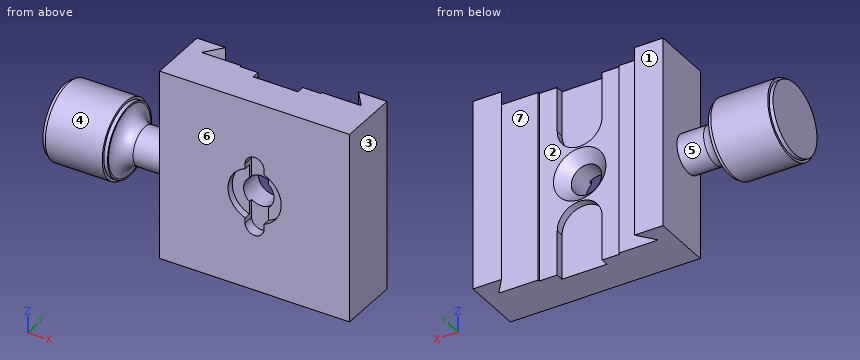
from build123d import *

# Parameters (mm, degrees)
SKETCH_1_R          = 5.9
EXTRUDE_1_DEPTH     = 8.94
SKETCH_1_4_R        = 4
EXTRUDE_2_DEPTH     = 11
SKETCH_1_5_W        = 14.4
SKETCH_1_5_H        = 50
EXTRUDE_3_DEPTH     = 16
CUT_EXTRUDE_1_DEPTH = 59.14636704
SKETCH_4_R          = 5
EXTRUDE_4_DEPTH     = 11
SKETCH_5_R          = 9.4
EXTRUDE_5_DEPTH     = 1
SKETCH_6_R          = 10.05
EXTRUDE_6_DEPTH     = 15
SKETCH_7_R          = 9.4
EXTRUDE_7_DEPTH     = 1
FILLET_1_R          = 4
CUT_EXTRUDE_3_DEPTH = 1.8
CUT_EXTRUDE_4_DEPTH = 2.8


with BuildPart() as part:
    # 草图1 → 凸台-拉伸1 (new body)
    with BuildSketch(Plane(origin=(0, 0, 0), x_dir=(1, 0, 0), z_dir=(0, 1, 0))):
        with BuildLine():
            Line((-5.9, -13.2), (-5.9, -25))
            Line((-5.9, -25), (5.9, -25))
            Line((5.9, -25), (5.9, -13.2))
            ThreePointArc((5.9, -13.2), (0, -19.1), (-5.9, -13.2))
        make_face()
        with Locations((0, -13.2)):
            Circle(SKETCH_1_R)
        with Locations((0, 13.2)):
            Circle(SKETCH_1_R)
        with BuildLine():
            Line((-5.9, 25), (-5.9, 13.2))
            ThreePointArc((-5.9, 13.2), (0, 19.1), (5.9, 13.2))
            Line((5.9, 13.2), (5.9, 25))
            Line((5.9, 25), (-5.9, 25))
        make_face()
    extrude(amount=EXTRUDE_1_DEPTH)

    # 草图1<4> → 凸台-拉伸2 (add)
    with BuildSketch(Plane(origin=(0, 0, 0), x_dir=(1, 0, 0), z_dir=(0, 1, 0))):
        with BuildLine():
            ThreePointArc((5.9, 13.2), (0, 7.3), (-5.9, 13.2))
            Line((-5.9, 13.2), (-5.9, 25))
            Line((-5.9, 25), (-10.6, 25))
            Line((-10.6, 25), (-10.6, -25))
            Line((-10.6, -25), (-5.9, -25))
            Line((-5.9, -25), (-5.9, -13.2))
            ThreePointArc((-5.9, -13.2), (0, -7.3), (5.9, -13.2))
            Line((5.9, -13.2), (5.9, -25))
            Line((5.9, -25), (10.6, -25))
            Line((10.6, -25), (10.6, 25))
            Line((10.6, 25), (5.9, 25))
            Line((5.9, 25), (5.9, 13.2))
        make_face()
        with Locations(Location((0, 0, 0), (0, 0, 270))):
            Circle(SKETCH_1_4_R, mode=Mode.SUBTRACT)
    extrude(amount=EXTRUDE_2_DEPTH)

    # 草图1<5> → 凸台-拉伸3 (add)
    with BuildSketch(Plane(origin=(0, 0, 0), x_dir=(1, 0, 0), z_dir=(0, 1, 0))):
        with Locations((17.8, 0)):
            Rectangle(SKETCH_1_5_W, SKETCH_1_5_H)
        with Locations((-17.8, 0)):
            Rectangle(SKETCH_1_5_W, SKETCH_1_5_H)
    extrude(amount=EXTRUDE_3_DEPTH)

    # 草图2 → 切除-拉伸1 (cut, through all)
    with BuildSketch(Plane.XY.offset(25)):
        Polygon((-17.5, 16), (-21, 11.5), (21, 11.5), (17.5, 16), align=None)
    extrude(amount=-CUT_EXTRUDE_1_DEPTH, mode=Mode.SUBTRACT)

    # 切除-拉伸2 cone 1 section (through the dimple's axis) → 切除-拉伸2 (revolve, cut)
    with BuildSketch(Plane(origin=(0, 11, 0), x_dir=(0, 0, 1), z_dir=(1, 0, 0))):
        Polygon((0, 0), (6.9, 0), (0, 6.9), align=None)
    revolve(axis=Axis((0, 11, 0), (0, -1, 0)), mode=Mode.SUBTRACT)

    # 草图4 → 凸台-拉伸4 (add)
    with BuildSketch(Plane.ZY.offset(25)):
        with Locations(Location((0, 5, 0), (0, 0, 270))):
            Circle(SKETCH_4_R)
    extrude(amount=EXTRUDE_4_DEPTH)

    # 草图5 → 凸台-拉伸5 (add)
    with BuildSketch(Plane.ZY.offset(36)):
        with Locations((0, 5)):
            Circle(SKETCH_5_R)
    extrude(amount=EXTRUDE_5_DEPTH)

    # 草图6 → 凸台-拉伸6 (add)
    with BuildSketch(Plane.ZY.offset(37)):
        with Locations((0, 5)):
            Circle(SKETCH_6_R)
    extrude(amount=EXTRUDE_6_DEPTH)

    # 草图7 → 凸台-拉伸7 (add)
    with BuildSketch(Plane.ZY.offset(52)):
        with Locations((0, 5)):
            Circle(SKETCH_7_R)
    extrude(amount=EXTRUDE_7_DEPTH)

    # 圆角1
    fillet_1_edges = [part.edges().sort_by_distance(p)[0] for p in [
        (-36, 10, 0),
    ]]
    fillet(fillet_1_edges, radius=FILLET_1_R)

    # 草图8 → 切除-拉伸3 (cut)
    with BuildSketch(Plane.XZ):
        with BuildLine():
            Line((-2.5, 3.122498999), (-2.5, 6.538348415))
            ThreePointArc((-2.5, 6.538348415), (-7, 0), (-2.5, -6.538348415))
            Line((-2.5, -6.538348415), (-2.5, -3.122498999))
            ThreePointArc((-2.5, -3.122498999), (-4, 0), (-2.5, 3.122498999))
        make_face()
        with BuildLine():
            ThreePointArc((7, 0), (5.766281297, 3.968626967), (2.5, 6.538348415))
            Line((2.5, 6.538348415), (2.5, 3.122498999))
            ThreePointArc((2.5, 3.122498999), (3.605551275, 1.732050808), (4, 0))
            ThreePointArc((4, 0), (3.605551275, -1.732050808), (2.5, -3.122498999))
            Line((2.5, -3.122498999), (2.5, -6.538348415))
            ThreePointArc((2.5, -6.538348415), (5.766281297, -3.968626967), (7, 0))
        make_face()
    extrude(amount=-CUT_EXTRUDE_3_DEPTH, mode=Mode.SUBTRACT)

    # 草图8<3> → 切除-拉伸4 (cut)
    with BuildSketch(Plane.XZ):
        with BuildLine():
            Line((2.5, 7.9), (2.5, -7.9))
            ThreePointArc((2.5, -7.9), (0, -10.4), (-2.5, -7.9))
            Line((-2.5, -7.9), (-2.5, 7.9))
            ThreePointArc((-2.5, 7.9), (0, 10.4), (2.5, 7.9))
        make_face()
    extrude(amount=-CUT_EXTRUDE_4_DEPTH, mode=Mode.SUBTRACT)


solid = part.part
CAD build for the part. Positions are in the model's coordinates, mm. Face numbers are marked on the shaded views. A direction names the side the tool comes from. Give positions to 0.01 mm unless a question says otherwise; leave off trailing zeros. Write each loop counter-clockwise with the first axis right and the second up, starting at its lowest first coordinate (ties: lowest second). Pieces come first, ordered by that corner, then holes. Notation, with made-up numbers: (-7, -2) -> (35, -2) arc R35 ccw to (35, 35) -> close; hole circle Ø2 at (29, 15). An arc over 180 degrees is marked (long way). Return JSON: item names as keys, results as strings.
Item 1: Band-saw the part on D-D (z = 11.5). List the corners of the cut face in (x, y), then the cut area to 3 significant figures.
Answer below:
{"outline": "(-25, 0) -> (25, 0) -> (25, 16) -> (17.5, 16) -> (21, 11.5) -> (10.6, 11.5) -> (10.6, 11) -> (5.65, 11) -> (5.65, 8.94) -> (-5.65, 8.94) -> (-5.65, 11) -> (-10.6, 11) -> (-10.6, 11.5) -> (-21, 11.5) -> (-17.5, 16) -> (-25, 16) -> close", "area": "593 mm2"}
Item 2: Tool access for the marked faces 4, 5, 6 and 7: list every direction of +Z, -Z, +X, -X, +Y, -Y with a clear straight run to the whole face (end or side of a thin tool).
Answer below:
{"face 4": "-X", "face 5": "none", "face 6": "+Z, -Z, +X, -Y", "face 7": "+Z, -Z"}
Item 3: Drill centre lines: probe 1 along X at (y, z) = (6, 0); probe 2 along Y at (x, z) = (5, 10); probe 3 along X at (y, z) = (0.5, 4.5). Where is each one in solid material? Low to high.
Answer below:
{"probe 1": "x = -53 to -4, 4 to 25", "probe 2": "y = 0 to 11", "probe 3": "x = -53 to -35.01, -25 to -5.36, 5.36 to 25"}
Item 4: Band-saw the part on C-C (x = -44.5). List the corners of the cut face in (y, z), then the cut area to 3 significant figures.
Answer below:
{"outline": "circle Ø20.1 at (5, 0)", "area": "317 mm2"}
Item 5: Band-saw the part on B-B (y = 5). List the corners of the cut face in (x, z).
Answer below:
{"outline": "(-53, -9.4) -> (-52, -9.4) -> (-52, -10.05) -> (-37, -10.05) -> (-37, -9.4) -> (-36, -9.4) -> (-36, -9) arc R4 cw to (-32, -5) -> (-25, -5) -> (-25, -25) -> (25, -25) -> (25, 25) -> (-25, 25) -> (-25, 5) -> (-32, 5) arc R4 cw to (-36, 9) -> (-36, 9.4) -> (-37, 9.4) -> (-37, 10.05) -> (-52, 10.05) -> (-52, 9.4) -> (-53, 9.4) -> close; hole circle Ø8 at (0, 0)"}
Item 6: Drop flat-ended pins along their axis: pin 1 (10.5 mm diameter, centred on x = 2, z = 2, fed in from +Y); pin 2 (1.5 mm diameter, centred on x = 0.5, z = 6, fed in from -Y); pin 3 (10.5 mm diameter, centred on x = 0, z = 0, fed in from -Y). Give the stop position or say it passes through.
Answer below:
{"pin 1": "stops at y = 11", "pin 2": "stops at y = 2.8", "pin 3": "stops at y = 1.8"}
Item 7: Band-saw the part on A-A (z = 18.5). List the corners of the cut face in (x, y).
Answer below:
{"outline": "(-25, 0) -> (25, 0) -> (25, 16) -> (17.5, 16) -> (21, 11.5) -> (10.6, 11.5) -> (10.6, 11) -> (5.9, 11) -> (5.9, 8.94) -> (-5.9, 8.94) -> (-5.9, 11) -> (-10.6, 11) -> (-10.6, 11.5) -> (-21, 11.5) -> (-17.5, 16) -> (-25, 16) -> close"}
Item 8: Two-plate mould, pull along X, no slides. Class the marked faces 1, 2 and 3: +X half, -X half, draft (parallel to the pull), parting line (faces both ways), or undercut.
Answer below:
{"face 1": "draft", "face 2": "undercut", "face 3": "+X half"}
